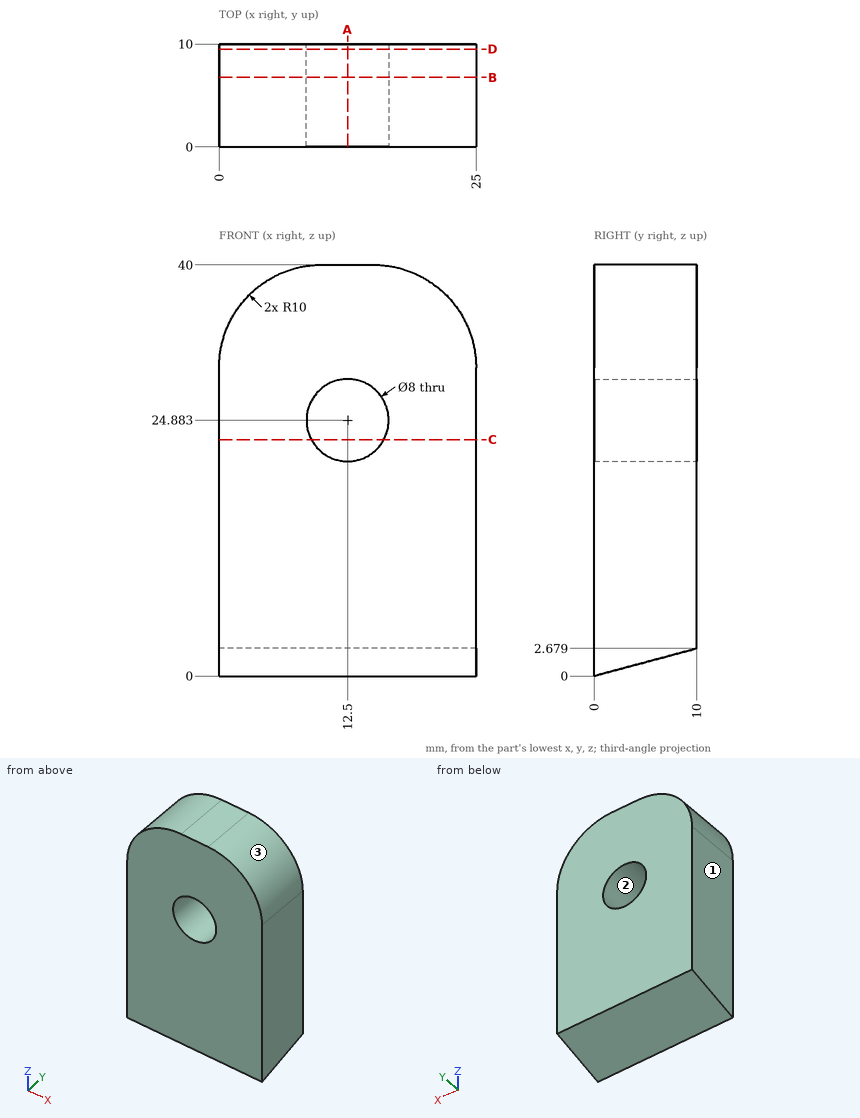
Design review of the part shown in the three views and the two pictorial views. Dimensions are in mm from the part's minimum x, y and z. Round coordinates to 2 decimals unless told otherwise and drop trailing zeros. Write each loop counter-clockwise with the first axis right and the second up, starting at its lowest first coordinate (ties: lowest second). Pieces come first, ordered by that corner, then holes. Notation, with made-up numbers: (80.5, 64.25) - (106.5, 64.25) arc R19 ccw to (106.5, 83.25) - close; hole circle Ø9 at (-22, 68.25). An arc over 180 degrees is marked (long way). Return JSON: item names as keys, results as strings. Group by question number.
Item 1: We need section B-B on y = 6.75. Write out the cut boundary in (x, z).
Item 2: We need section C-C on z = 23. Write out the cut boundary in (x, y).
Item 3: The part is to be moulded in two halves that separate along Z. For the marked faces 1, 2 and 3, say which applies: pulls with the +Z half, pulls with the -Z half, needs draft (parallel to the pull), parting line crosses it, or undercut.
Item 4: Insertion check: P1, Ø7, axis at x = 12.5, z = 24.88, coming from the -Y side; P2, Ø5, axis at y = 4.5, z = 35, coming from the -X side. Each pin has a flat end and moves straight along its axis. Give the tip position at first contact, or say it passes through.
Item 5: We need section D-D on y = 9.5. Write out the cut boundary in (x, z) (1 decimal).
Item 6: For probe 1 along Z at (x, y) = (11, 7) (1 decimal); probe 2 along Z at (x, y) = (12.5, 5.75); probe 3 along X at (y, z) = (8.75, 27) (1 decimal), list the stretches that pass through material, from the lowest coordinate up. Write a range as [from, to].
Item 7: We need section A-A on x = 12.5. Write out the cut boundary in (y, z), and give its area (3 significant figures).
Model answer:
{
 "1": {"outline": "(0, 1.81) - (25, 1.81) - (25, 30) arc R10 ccw to (15, 40) - (10, 40) arc R10 ccw to (0, 30) - close; hole circle Ø8 at (12.5, 24.88)"},
 "2": {"outline": "(0, 0) - (8.97, 0) - (8.97, 10) - (0, 10) - close; (16.03, 0) - (25, 0) - (25, 10) - (16.03, 10) - close"},
 "3": {"face 1": "needs draft", "face 2": "undercut", "face 3": "pulls with the +Z half"},
 "4": {"P1": "passes through", "P2": "stops at x = 0.32"},
 "5": {"outline": "(0, 2.5) - (25, 2.5) - (25, 30) arc R10 ccw to (15, 40) - (10, 40) arc R10 ccw to (0, 30) - close; hole circle Ø8 at (12.5, 24.9)"},
 "6": {"probe 1": "z = [1.9, 21.2], [28.6, 40]", "probe 2": "z = [1.54, 20.88], [28.88, 40]", "probe 3": "x = [0, 9.1], [15.9, 25]"},
 "7": {"outline": "(0, 0) - (10, 2.68) - (10, 20.88) - (0, 20.88) - close; (0, 28.88) - (10, 28.88) - (10, 40) - (0, 40) - close", "area": "307 mm²"}
}
